Can you work these out from the drawing? Everything is in mm from the part's minimum corner. Give positions to 0.01 mm unless a question says otherwise; leave off trailing zeros. Order: outer loops, then holes, each group sorted by start corner. A loop starts at its lowest first (then second) coordinate and runs counter-clockwise, first axis right, second up. Notation, with made-up numbers: M -3.75,-13.5 L 15.25,-13.5 A29 cw 15.25,11.5 Z; hole C -32,47 d10. An arc over 180 degrees is marked long. Answer as a JSON object with one key per item and string values.
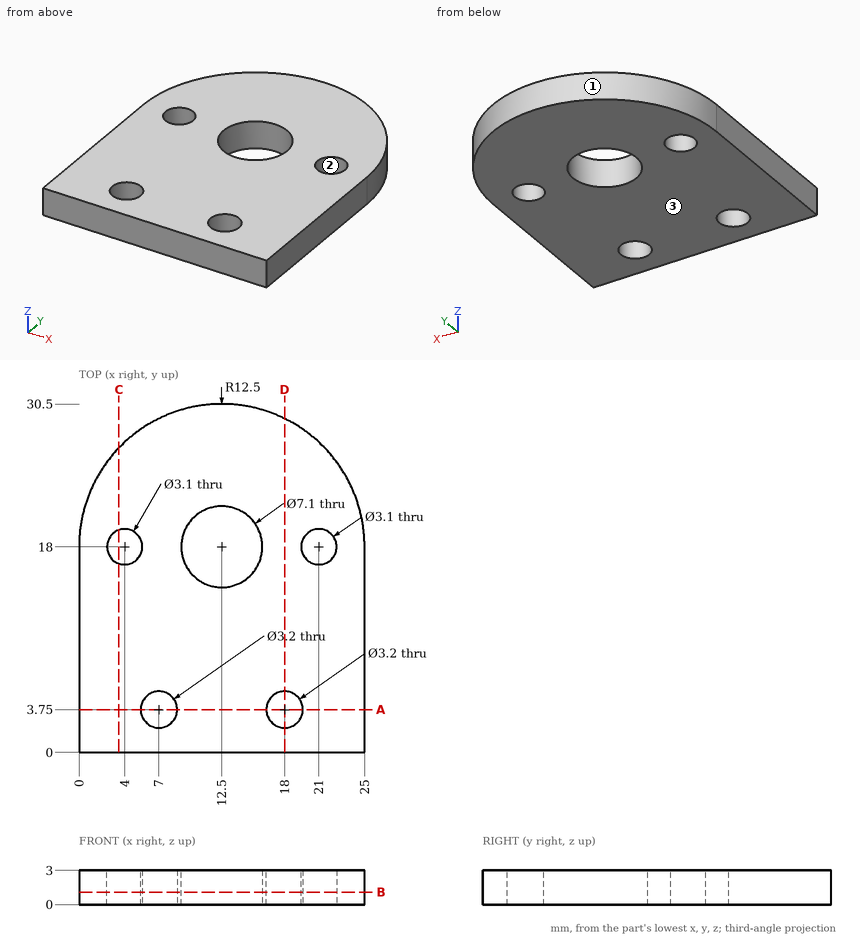
1) I'm going to push flat-ended pins straight in: pin 1 Ø5.5 at (x, y) = (12.5, 18) entering from +Z; pin 2 Ø1.5 at (y, z) = (23.5, 0.5) entering from +X. Where does each tip first touch, or does it pass through?
Results found:
{"pin 1": "passes through", "pin 2": "stops at x = 24.06"}
2) I want a section at A-A on y = 3.75. Write out the boundary of the cut face in (x, z), and give its area (3 significant figures).
Results found:
{"outline": "M 0,0 L 5.4,0 L 5.4,3 L 0,3 Z; M 8.6,0 L 16.4,0 L 16.4,3 L 8.6,3 Z; M 19.6,0 L 25,0 L 25,3 L 19.6,3 Z", "area": "55.8 mm²"}
3) I need wall thicknesses on L1, parallel to Y at x = 7, z = 1.35; L2, parallel to Y at x = 4, z = 0.6; L3, parallel to X at y = 3, z = 1.05. Which ranges of each line are inside material? Lowest first, please.
Results found:
{"L1": "y = 0 to 2.15, 5.35 to 29.22", "L2": "y = 0 to 16.45, 19.55 to 27.17", "L3": "x = 0 to 5.59, 8.41 to 16.59, 19.41 to 25"}
4) I want a section at D-D on x = 18. Write out the boundary of the cut face in (y, z), and give its area (3 significant figures).
Results found:
{"outline": "M 0,0 L 2.15,0 L 2.15,3 L 0,3 Z; M 5.35,0 L 29.22,0 L 29.22,3 L 5.35,3 Z", "area": "78.1 mm²"}
5) Thinking about a two-plate mould opening in Y: for the marked faces 1, 2 and 3, which applies, pulls with the +Y half, pulls with the -Y half, needs draft (parallel to the pull), parting line crosses it, or undercut?
Results found:
{"face 1": "pulls with the +Y half", "face 2": "undercut", "face 3": "needs draft"}
6) I want a section at B-B on z = 1.1. Write out the boundary of the cut face in (x, y).
Results found:
{"outline": "M 0,0 L 25,0 L 25,18 A12.5 ccw 0,18 Z; hole C 4,18 d3.1; hole C 7,3.75 d3.2; hole C 12.5,18 d7.1; hole C 18,3.75 d3.2; hole C 21,18 d3.1"}
7) I want a section at C-C on x = 3.5. Write out the boundary of the cut face in (y, z).
Results found:
{"outline": "M 0,0 L 16.53,0 L 16.53,3 L 0,3 Z; M 19.47,0 L 26.67,0 L 26.67,3 L 19.47,3 Z"}
